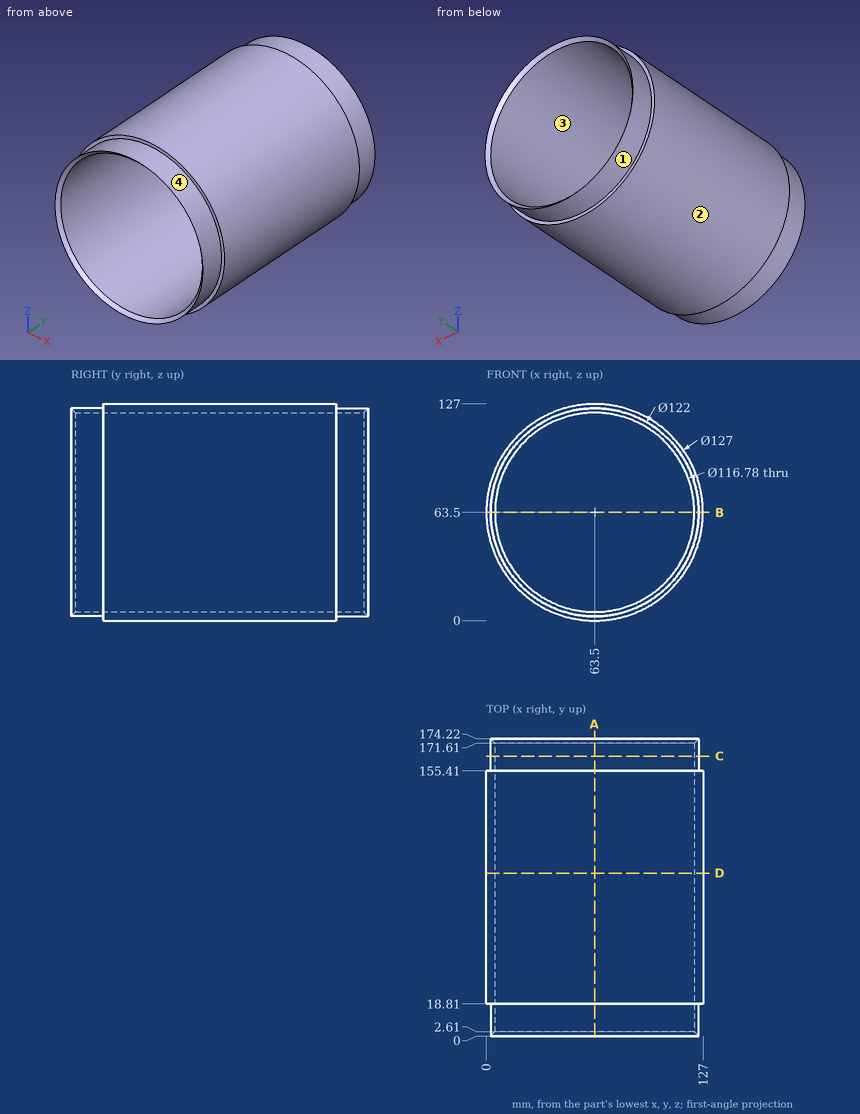
Geometry: see drawing. Coordinates: mm, zero at the bounding-box minimum. A direction names the side the tool comes from. Give positions to 0.01 mm unless a question says otherwise; leave off trailing zeros. Loops run counter-clockwise (first coordinate to the right, second up) from the corner with the lowest first, then second, coordinate; pieces in that order, holes last. Notation, with made-up numbers: M 4.25,2 L 62.25,2 A21 ccw 62.25,22 Z; hole C 34,49 d9. An arc over 180 degrees is marked long. Answer as CSV lines item,"result". Start each with the question number.
1. Line query: L1, parallel to Z at x = 63.5, y = 129.5; L2, parallel to Z at x = 96.5, y = 141.5. Output: solid intervals per line, ascending.
2. Reachability of the marked faces 1 and 2 from +Z, -Z, +X, -X, +Y, -Y: full face, straight path, thin tool, end or side. Return the list, or none.
3. Pin query (flat end, axial travel): P1, Ø2, axis at x = 57.5, y = 152.5, coming from the +Z side; P2, Ø10, axis at x = 62.5, y = 134, coming from the +Z side; P3, Ø8, axis at x = 19.5, y = 75, coming from the +Z side. Return the tip coordinate at first contact, or that it passes through.
4. Section D-D on y = 95.5. Return loops of the section in (x, z).
5. Section C-C on y = 164. Return loops of the section in (x, z), plus the area to 3 significant figures.
6. Section B-B on z = 63.5. Return loops of the section in (x, y).
7. Section A-A on x = 63.5. Return loops of the section in (y, z).
8. Pull-direction query (X, two-part tool) for the marked faces 3 and 4; classes: released by +X, released by -X, zero draft, split by the parting line, or undercut.
Computed values:
1,L1,"z = 0 to 5.11, 121.89 to 127"
1,L2,"z = 9.25 to 15.33, 111.67 to 117.75"
2,face 1,"+Y"
2,face 2,"+Y, -Y"
3,P1,"stops at z = 126.8"
3,P2,"stops at z = 127"
3,P3,"stops at z = 112.82"
4,outline,"C 63.5,63.5 d127; hole C 63.5,63.5 d116.78"
5,outline,"C 63.5,63.5 d122; hole C 63.5,63.5 d116.78"
5,area,"979 mm²"
6,outline,"M 0,18.81 L 2.5,18.81 L 2.5,0 L 5.11,2.61 L 5.11,171.61 L 2.5,174.22 L 2.5,155.41 L 0,155.41 Z; M 121.89,2.61 L 124.5,0 L 124.5,18.81 L 127,18.81 L 127,155.41 L 124.5,155.41 L 124.5,174.22 L 121.89,171.61 Z"
7,outline,"M 0,2.5 L 18.81,2.5 L 18.81,0 L 155.41,0 L 155.41,2.5 L 174.22,2.5 L 171.61,5.11 L 2.61,5.11 Z; M 0,124.5 L 2.61,121.89 L 171.61,121.89 L 174.22,124.5 L 155.41,124.5 L 155.41,127 L 18.81,127 L 18.81,124.5 Z"
8,face 3,"undercut"
8,face 4,"split by the parting line"
